from build123d import *

# Parameters (mm, degrees)
BOSS_EXTRUDE1_DEPTH     = 12.7
BOSS_EXTRUDE2_DEPTH     = 1.016
CUT_EXTRUDE2_DEPTH      = 0.254
CUT_EXTRUDE2_DEPTH_BACK = 0.254
SKETCH8_R               = 3.782150116
SKETCH8_R_2             = 0.533461952
SKETCH7_R               = 5.190476509
CUT_EXTRUDE3_DEPTH      = 0.254
CUT_EXTRUDE5_DEPTH      = 0.254
SKETCH13_R              = 2.893074104
CUT_EXTRUDE7_DEPTH      = 11.43
CUT_EXTRUDE8_DEPTH      = 7.62
BOSS_EXTRUDE3_DEPTH     = 0.254


with BuildPart() as part:
    # Sketch2 → Boss-Extrude1 (new body)
    with BuildSketch(Plane(origin=(0, 0, 0), x_dir=(1, 0, 0), z_dir=(0, 1, 0))):
        with BuildLine():
            Line((23.304511321, 59.876164022), (-40.195488679, 59.876164022))
            ThreePointArc((-40.195488679, 59.876164022), (-43.787591127, 58.388266471), (-45.275488679, 54.796164022))
            Line((-45.275488679, 54.796164022), (-45.275488679, -72.203835978))
            ThreePointArc((-45.275488679, -72.203835978), (-43.787591127, -75.795938426), (-40.195488679, -77.283835978))
            Line((-40.195488679, -77.283835978), (23.304511321, -77.283835978))
            ThreePointArc((23.304511321, -77.283835978), (26.89661377, -75.795938426), (28.384511321, -72.203835978))
            Line((28.384511321, -72.203835978), (28.384511321, 54.796164022))
            ThreePointArc((28.384511321, 54.796164022), (26.89661377, 58.388266471), (23.304511321, 59.876164022))
        make_face()
    extrude(amount=BOSS_EXTRUDE1_DEPTH)

    # Sketch5 → Boss-Extrude2 (add)
    with BuildSketch(Plane(origin=(0, 0, 0), x_dir=(-1, 0, 0), z_dir=(0, -1, 0))):
        with BuildLine():
            Line((1.259403459, 20.324166162), (1.259403459, 47.177431984))
            ThreePointArc((1.259403459, 47.177431984), (8.256381173, 54.174409699), (15.253358888, 47.177431984))
            Line((15.253358888, 47.177431984), (15.253358888, 20.324166162))
            ThreePointArc((15.253358888, 20.324166162), (8.256381173, 13.327188447), (1.259403459, 20.324166162))
        make_face()
    extrude(amount=BOSS_EXTRUDE2_DEPTH)

    # Sketch8 → Cut-Extrude2 (cut, two sides: drawn at the far end of the back side and taken through both)
    with BuildSketch(Plane(origin=(0, -1.016, 0), x_dir=(-1, 0, 0), z_dir=(0, -1, 0)).offset(-CUT_EXTRUDE2_DEPTH_BACK)):
        with Locations(Location((8.256381173, 29.871883473, 0), (0, 0, 90))):
            Circle(SKETCH8_R)
        with Locations(Location((8.256381173, 20.324166162, 0), (0, 0, 90))):
            Circle(SKETCH8_R_2)
    extrude(amount=CUT_EXTRUDE2_DEPTH + CUT_EXTRUDE2_DEPTH_BACK, mode=Mode.SUBTRACT)

    # Sketch7 → Cut-Extrude3 (cut)
    with BuildSketch(Plane(origin=(0, -1.016, 0), x_dir=(-1, 0, 0), z_dir=(0, -1, 0))):
        with Locations(Location((8.256381173, 45.395398439, 0), (0, 0, 90))):
            Circle(SKETCH7_R)
    extrude(amount=-CUT_EXTRUDE3_DEPTH, mode=Mode.SUBTRACT)

    # Sketch10 → Cut-Extrude5 (cut)
    with BuildSketch(Plane(origin=(0, 12.7, 0), x_dir=(1, 0, 0), z_dir=(0, 1, 0))):
        with BuildLine():
            Line((-22.628551613, 52.094227135), (1.577209128, 52.094227135))
            ThreePointArc((1.577209128, 52.094227135), (3.27917668, 50.392259583), (1.577209128, 48.690292031))
            Line((1.577209128, 48.690292031), (-22.628551613, 48.690292031))
            ThreePointArc((-22.628551613, 48.690292031), (-24.330519166, 50.392259583), (-22.628551613, 52.094227135))
        make_face()
    extrude(amount=-CUT_EXTRUDE5_DEPTH, mode=Mode.SUBTRACT)

    # Sketch13 → Cut-Extrude7 (cut)
    with BuildSketch(Plane(origin=(0, 0, -59.876164022), x_dir=(-1, 0, 0), z_dir=(0, 0, -1))):
        with Locations((26.098165184, 2.993499928)):
            Circle(SKETCH13_R)
    extrude(amount=-CUT_EXTRUDE7_DEPTH, mode=Mode.SUBTRACT)

    # Sketch14 → Cut-Extrude8 (cut)
    with BuildSketch(Plane(origin=(0, 0, -59.876164022), x_dir=(-1, 0, 0), z_dir=(0, 0, -1))):
        with BuildLine():
            Line((4.185340578, 5.307383364), (13.751795184, 5.307383364))
            ThreePointArc((13.751795184, 5.307383364), (16.080302046, 2.978876501), (13.751795184, 0.650369639))
            Line((13.751795184, 0.650369639), (4.185340578, 0.650369639))
            ThreePointArc((4.185340578, 0.650369639), (1.856833715, 2.978876501), (4.185340578, 5.307383364))
        make_face()
        with BuildLine():
            Line((4.185340578, 3.812772213), (13.751795184, 3.812772213))
            ThreePointArc((13.751795184, 3.812772213), (14.585690896, 2.978876501), (13.751795184, 2.144980789))
            Line((13.751795184, 2.144980789), (4.185340578, 2.144980789))
            ThreePointArc((4.185340578, 2.144980789), (3.351444866, 2.978876501), (4.185340578, 3.812772213))
        make_face(mode=Mode.SUBTRACT)
    extrude(amount=-CUT_EXTRUDE8_DEPTH, mode=Mode.SUBTRACT)

    # Sketch16 → Boss-Extrude3 (add)
    with BuildSketch(Plane(origin=(28.384511321, 0, 0), x_dir=(0, 0, -1), z_dir=(1, 0, 0))):
        with BuildLine():
            Line((1.812614233, 5.138816206), (22.282032337, 5.138816206))
            ThreePointArc((22.282032337, 5.138816206), (23.477323285, 3.943525258), (22.282032337, 2.748234309))
            Line((22.282032337, 2.748234309), (1.812614233, 2.748234309))
            ThreePointArc((1.812614233, 2.748234309), (0.617323285, 3.943525258), (1.812614233, 5.138816206))
        make_face()
        with BuildLine():
            Line((-14.226212683, 5.138811158), (-5.261520474, 5.138811158))
            ThreePointArc((-5.261520474, 5.138811158), (-4.066234574, 3.943525258), (-5.261520474, 2.748239358))
            Line((-5.261520474, 2.748239358), (-14.226212683, 2.748239358))
            ThreePointArc((-14.226212683, 2.748239358), (-15.421498583, 3.943525258), (-14.226212683, 5.138811158))
        make_face()
    extrude(amount=BOSS_EXTRUDE3_DEPTH)


solid = part.part
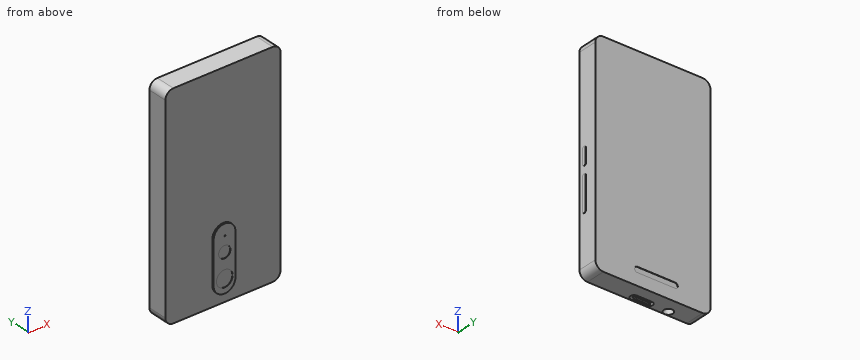
CAD build for the part. Positions are in the model's coordinates, mm. Coordinates: 2 decimals unless noted, no trailing zeros. Order: outer loops, then holes, each group sorted by start corner. A loop starts at its lowest first (then second) coordinate and runs counter-clockwise, first axis right, second up. Notation, with made-up numbers: (57.25, 82.5) -> (80.25, 82.5) arc R15 ccw to (80.25, 103.5) -> close; hole circle Ø8 at (80, 3.5). An arc over 180 degrees is marked (long way). Answer in a Markdown table with one row per item.
1) Band-saw the part on A-A (z = -36). List the corners of the cut face in (x, y).
Check values:
| item | result |
|---|---|
| outline | (-45.28, 0) -> (-15.25, 0) -> (-15.25, -1.02) -> (-1.26, -1.02) -> (-1.26, 0) -> (28.38, 0) -> (28.38, 12.7) -> (-45.28, 12.7) -> close |
2) Flat gauge pins, fed straight in: P1, Ø1.5, axis at x = 11, z = 60, coming from the -Y side; P2, Ø2, axis at y = 6.5, z = 28, coming from the +X side; P3, Ø2.5, axis at x = -8.5, z = -28.5, coming from the -Y side. Where does each tip first touch, or does it go through?
Check values:
| item | result |
|---|---|
| P1 | y = 0 |
| P2 | x = 28.38 |
| P3 | y = -0.76 |
3) Band-saw the part on D-D (z = 39). List the corners of the cut face in (x, y), and give its area (3 significant figures).
Check values:
| item | result |
|---|---|
| outline | (-45.28, 0) -> (28.38, 0) -> (28.38, 12.7) -> (-45.28, 12.7) -> close |
| area | 935 mm2 |
4) Band-saw the part on B-B (x = 9). List the corners of the cut face in (y, z).
Check values:
| item | result |
|---|---|
| outline | (0, -59.88) -> (12.7, -59.88) -> (12.7, 77.28) -> (0, 77.28) -> close |
5) Band-saw the part on C-C (z = -9.5). List the corners of the cut face in (x, y), and give its area (3 significant figures).
Check values:
| item | result |
|---|---|
| outline | (-45.28, 0) -> (28.38, 0) -> (28.38, 2.75) -> (28.64, 2.75) -> (28.64, 5.14) -> (28.38, 5.14) -> (28.38, 12.7) -> (-45.28, 12.7) -> close |
| area | 936 mm2 |
6) Drill centre lines: line 1 (X direction, y = 11, z = 53); line 2 (Y direction, x = -35, z = -40); line 3 (Y direction, x = -5, z = -44.5). Where is each one in solid material? Low to high.
Check values:
| item | result |
|---|---|
| line 1 | -45.28 to 28.38 |
| line 2 | 0 to 12.7 |
| line 3 | -0.76 to 12.7 |
